Geometry: final body of the model. Coordinates: model frame, mm. A direction names the side the tool comes from. Coordinates: 2 decimals unless noted, no trailing zeros. Order: outer loops, then holes, each group sorted by start corner. A loop starts at its lowest first (then second) coordinate and runs counter-clockwise, first axis right, second up. Notation, with made-up numbers: M -19,-4.75 L 25,-4.75 A13 cw 25,-0.75 Z; hole C 69.25,-7 d3. An arc over 180 degrees is marked long. One line per question, with ' | ' between items.
from build123d import *

# Parameters (mm, degrees)
F0_R     = 2.5
F0_R_2   = 3.5
F1_DEPTH = 3


# Not quite as in the source:
# - a fillet or chamfer that OpenCascade refuses, or shapes differently, is made with other operations: its cross-section is extruded or revolved along the edge and cut away or added


with BuildPart() as f1:
    # F0 (on Front) → F1 (new body)
    with BuildSketch(Plane.XZ):
        with BuildLine():
            ThreePointArc((8.6618165432, -19.5581924259), (14.9578845034, -21.7890529471), (18.4448225733, -27.4862867778))
            ThreePointArc((18.4448225733, -27.4862867778), (33.9501260505, -36.3938374492), (41.0935207185, -20.0008265146))
            ThreePointArc((41.0935207185, -20.0008265146), (40.4143456003, -17.9668557736), (40.1844298095, -15.8348486101))
            Line((40.1844298095, -15.8348486101), (40.1844298095, 15.8348486101))
            ThreePointArc((40.1844298095, 15.8348486101), (40.4143456003, 17.9668557736), (41.0935207185, 20.0008265146))
            ThreePointArc((41.0935207185, 20.0008265146), (34.0564016131, 36.3581615745), (18.4933227899, 27.7051832948))
            ThreePointArc((18.4933227899, 27.7051832948), (14.9739484465, 22.1318851219), (8.750733607, 19.9595027072))
            Line((8.750733607, 19.9595027072), (-32, 19.9595027072))
            ThreePointArc((-32, 19.9595027072), (-37.6568542495, 17.6163569566), (-40, 11.9595027072))
            Line((-40, 11.9595027072), (-40, -12))
            ThreePointArc((-40, -12), (-37.5106423232, -17.3691502038), (-32.0122089369, -19.5581924259))
            Line((-32.0122089369, -19.5581924259), (8.6618165432, -19.5581924259))
        make_face()
        with Locations((-30, -10)):
            Circle(F0_R, mode=Mode.SUBTRACT)
        with Locations((30.1844298095, -25)):
            Circle(F0_R, mode=Mode.SUBTRACT)
        with Locations((30.1844298095, -10)):
            Circle(F0_R, mode=Mode.SUBTRACT)
        with Locations((-30, 10)):
            Circle(F0_R_2, mode=Mode.SUBTRACT)
        with Locations((30.1844298095, 10)):
            Circle(F0_R, mode=Mode.SUBTRACT)
        with Locations((30.1844298095, 25)):
            Circle(F0_R, mode=Mode.SUBTRACT)
    extrude(amount=F1_DEPTH)

    # F2: chamfer of 3.5 on 3 edges, made by hand

    # F2_s1 → F2_t2 (revolve, cut)
    with BuildSketch(Plane.XY.offset(10)):
        Polygon((32.6844298095, -3.5), (36.1844298095, 0), (32.6844298095, 0), align=None)
    revolve(axis=Axis((30.1844298095, 0, 10), (0, -1, 0)), mode=Mode.SUBTRACT)

    # F2_s3 → F2_t4 (revolve, cut)
    with BuildSketch(Plane.XY.offset(-10)):
        Polygon((32.6844298095, -3.5), (36.1844298095, 0), (32.6844298095, 0), align=None)
    revolve(axis=Axis((30.1844298095, 0, -10), (0, -1, 0)), mode=Mode.SUBTRACT)

    # F2_s5 → F2_t6 (revolve, cut)
    with BuildSketch(Plane.XY.offset(-10)):
        Polygon((-27.5, -3.5), (-24, 0), (-27.5, 0), align=None)
    revolve(axis=Axis((-30, 0, -10), (0, -1, 0)), mode=Mode.SUBTRACT)


solid = f1.part
1. Section D-D, the plane z = -25. Output: boundary loops of the cut face in (x, y), and give its area (3 significant figures).
Response values:
outline: M 17.56,-3 L 27.68,-3 L 27.68,0 L 17.56,0 Z; M 32.68,-3 L 42.18,-3 L 42.18,0 L 32.68,0 Z | area: 58.9 mm^2
2. Access query for faces 1 (the face through (-11, -1, 19.96)), 2 (the face through (-12, -1, -19.558)), 3 (the face through (40.184, -1, 0)). Directions: +Z, -Z, +X, -X, +Y, -Y. A direction counts if a zero-diameter tool reaches every point of the face in a straight line with its end or side. Return the directions, or none.
Response values:
face 1: +Z, -X, +Y, -Y | face 2: -Z, -X, +Y, -Y | face 3: +X, +Y, -Y
3. Section A-A, the plane x = -30. Output: boundary loops of the cut face in (y, z), and give its area (3 significant figures).
Response values:
outline: M -3,-19.56 L 0,-19.56 L 0,-16 L -3,-13 Z; M -3,-7 L 0,-4 L 0,6.5 L -3,6.5 Z; M -3,13.5 L 0,13.5 L 0,19.96 L -3,19.96 Z | area: 70.6 mm^2
4. Section B-B, the plane z = 10. Output: boundary loops of the cut face in (x, y).
Response values:
outline: M -40,-3 L -33.5,-3 L -33.5,0 L -40,0 Z; M -26.5,-3 L 27.18,-3 L 24.18,0 L -26.5,0 Z; M 33.18,-3 L 40.18,-3 L 40.18,0 L 36.18,0 Z
5. Section C-C, the plane y = -1.4. Output: boundary loops of the cut face in (x, z), and give its area (3 significant figures).
Response values:
outline: M -40,-12 A8 ccw -32.01,-19.56 L 8.66,-19.56 A10 cw 18.44,-27.49 A12 ccw long 41.09,-20 A10 cw 40.18,-15.83 L 40.18,15.83 A10 cw 41.09,20 A12 ccw long 18.49,27.71 A10 cw 8.75,19.96 L -32,19.96 A8 ccw -40,11.96 Z; hole C -30,-10 d9.2; hole C -30,10 d7; hole C 30.18,-10 d9.2; hole C 30.18,10 d9.2; hole C 30.18,-25 d5; hole C 30.18,25 d5 | area: 3,600 mm^2
6. Pin query (flat end, axial travel): P1, Ø0.9, axis at y = -1, z = -7, coming from the +X side; P2, Ø1, axis at x = -0.5, y = -1.5, coming from the +Z side. Return the tip coordinate at first contact, or that it passes through.
Response values:
P1: stops at x = 40.18 | P2: stops at z = 19.96
7. Material intervals for line 1 (Z direction, x = 27, y = -2); line 2 (Z direction, x = -30, y = -0.8); line 3 (Z direction, x = -25, y = -1.6), sorted ascending. Write a range as [from, to].
Response values:
line 1: z = [-36.57, -12.42], [-7.58, 7.58], [12.42, 36.57] | line 2: z = [-19.56, -15.2], [-4.8, 6.5], [13.5, 19.96] | line 3: z = [-19.56, 19.96]
8. Draft query along Z for faces 4 (the face through (40.4, -1.5, 17.9)), 5 (the face through (-37.59, -1.48, 17.68)), 6 (the face through (-37.57, -1.48, -17.31)). Return one class per face: pulls with the +Z half, pulls with the -Z half, needs draft (parallel to the pull), parting line crosses it, or undercut.
Response values:
face 4: undercut | face 5: pulls with the +Z half | face 6: pulls with the -Z half
